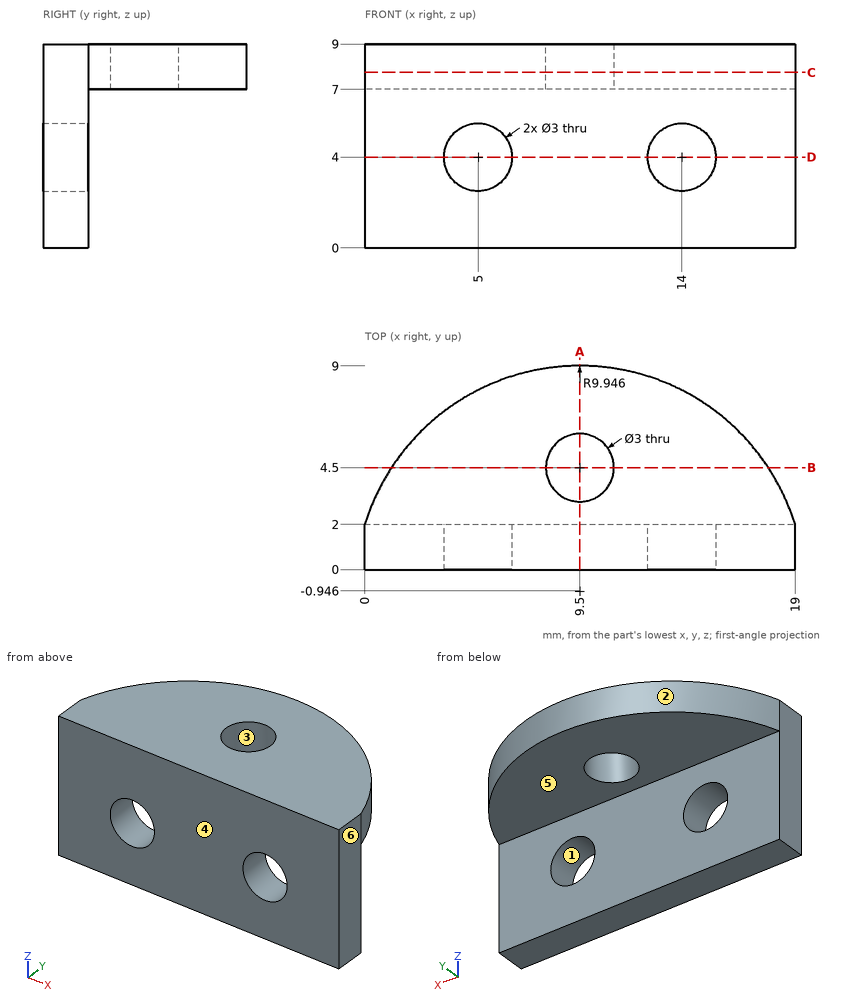
Job drawing, mm, ordinate dimensions from the low corner. One solid piece. A direction names the side the tool comes from. Give positions to 0.01 mm unless a question says otherwise; leave off trailing zeros. Order: outer loops, then holes, each group sorted by start corner. A loop starts at its lowest first (then second) coordinate and runs counter-clockwise, first axis right, second up. Notation, with made-up numbers: M -37,16.25 L -15,16.25 A12 ccw -15,35.25 Z; hole C -2.75,-23 d1. An arc over 180 degrees is marked long. Return JSON: item names as keys, results as strings.
Q1. Flat gauge pins, fed straight in: pin 1 (2 mm diameter, centred on y = 4.5, z = 1.5, fed in from -X); pin 2 (4 mm diameter, centred on x = 5, z = 4, fed in from +Y); pin 3 (4 mm diameter, centred on x = 9.5, y = 4.5, fed in from -Z). Where does each tip first touch, or does it go through?
Answer list:
{"pin 1": "passes through", "pin 2": "stops at y = 2", "pin 3": "stops at z = 7"}
Q2. Band-saw the part on C-C (z = 7.75). Give the cut face in (x, y).
Answer list:
{"outline": "M 0,0 L 19,0 L 19,2 A9.95 ccw 0,2 Z; hole C 9.5,4.5 d3"}
Q3. Two-plate mould, pull along X, no slides. Class the marked faces 1, 2, 3 and 4: pulls with the +X half, pulls with the -X half, needs draft (parallel to the pull), parting line crosses it, or undercut.
Answer list:
{"face 1": "undercut", "face 2": "parting line crosses it", "face 3": "undercut", "face 4": "needs draft"}
Q4. Band-saw the part on D-D (z = 4). Give the cut face in (x, y).
Answer list:
{"outline": "M 0,0 L 3.5,0 L 3.5,2 L 0,2 Z; M 6.5,0 L 12.5,0 L 12.5,2 L 6.5,2 Z; M 15.5,0 L 19,0 L 19,2 L 15.5,2 Z"}
Q5. 3-axis set-ups, long thin cutter, end or side, ignore diameter. For the marked faces 5 and 6: which of +Z, -Z, +X, -X, +Y, -Y reach the whole face in a straight line?
Answer list:
{"face 5": "-Z, +X, -X, +Y", "face 6": "+Z, -Z, +X, +Y, -Y"}
Q6. Band-saw the part on A-A (x = 9.5). Give the cut face in (y, z).
Answer list:
{"outline": "M 0,0 L 2,0 L 2,7 L 3,7 L 3,9 L 0,9 Z; M 6,7 L 9,7 L 9,9 L 6,9 Z"}
Q7. Wall check: probe 1 along X at (y, z) = (1, 4); probe 2 along Z at (x, y) = (5, 1.15); probe 3 along Y at (x, z) = (9.5, 8.1). Give the ranges that are in metal, low to high. Write a range as from..to.
Answer list:
{"probe 1": "x = 0..3.5, 6.5..12.5, 15.5..19", "probe 2": "z = 0..2.5, 5.5..9", "probe 3": "y = 0..3, 6..9"}
Q8. Band-saw the part on B-B (y = 4.5). Give the cut face in (x, z).
Answer list:
{"outline": "M 1.18,7 L 8,7 L 8,9 L 1.18,9 Z; M 11,7 L 17.82,7 L 17.82,9 L 11,9 Z"}
